Geometry check sheet. Reference: the model listing, model coordinates, mm. A direction names the side the tool comes from. Round coordinates to 2 decimals unless told otherwise and drop trailing zeros. Write each loop counter-clockwise with the first axis right and the second up, starting at its lowest first coordinate (ties: lowest second). Pieces come first, ordered by that corner, then holes. Notation, with made-up numbers: M 78,80.5 L 115,80.5 A13 cw 115,91.5 Z; hole C 3,-38.5 d10. An arc over 180 degrees is marked long. Put each result on its own line as item: value. Start each with the question number.
(1) Material ranges on probe 1 along Y at (x, z) = (-19.5, 26.5); probe 2 along Y at (x, z) = (8.5, 14.5); probe 3 along Z at (x, y) = (-68, 3), recorded low to high.
(2) Section check C-C on y = 19.5. Record the cut outline in (x, z).
(3) Section check D-D on y = -3.5. Record the cut outline in (x, z), then the cut area to 3 significant figures.
(4) Gauge pin test, flat ends, axial feed: pin 1 (9 mm diameter, centred on x = -21, y = -0.5, fed in from +Z); pin 2 (19 mm diameter, centred on x = -26, z = 25, fed in from -Y); pin 3 (13.5 mm diameter, centred on x = 30, y = -71, fed in from +Z). Record the tip position at first contact, or that the pin passes through.
(5) Section check B-B on x = 63. Record the cut outline in (y, z).
(6) Tool access check on faces 1 (the flat face through (-1, -53, 32.545)), 2 (the flat face through (2, -68, 15.158)), 3 (the flat face through (2, 4.999, 23)). Record the directions out of +Z, -Z, +X, -X, +Y, -Y that give a thin tool (end or side, any length) a straight path to the whole face; none if there is none.
(7) Section check A-A on z = 19.5. Record the cut outline in (x, y), then the cut area to 3 significant figures.
from build123d import *

# Parameters (mm, degrees)
F0_W     = 153.3627957106
F0_H     = 90.0560617447
F1_DEPTH = 76.6826
F2_W     = 17.0374948467
F2_H     = 17.3870613798
F2_W_2   = 19.1703476012
F2_H_2   = 18.2787058875
F2_W_3   = 17.8328882903
F2_W_4   = 17.3870567232
F2_H_3   = 19.1703503951
F2_W_5   = 17.8328789771
F2_H_4   = 17.832884565
F3_DEPTH = 228.6


with BuildPart() as f1:
    # F0 (on Front) → F1 (new body, symmetric)
    with BuildSketch(Plane.XZ):
        with Locations((0.4458203912, -12.4830156565)):
            Rectangle(F0_W, F0_H)
    extrude(amount=F1_DEPTH, both=True)

    # F2 (on face) → F3 (cut)
    with BuildSketch(Plane.YZ.offset(77.1272182465)):
        with Locations((-68.1638525767, 23.8514845259)):
            Rectangle(F2_W, F2_H)
        with Locations((-35.7936229557, 23.4056622721)):
            Rectangle(F2_W_2, F2_H_2)
        with Locations((-3.9173448458, 23.4056622721)):
            Rectangle(F2_W_3, F2_H_2)
        with Locations((26.1756433174, 22.9598400183)):
            Rectangle(F2_W_4, F2_H_3)
        with Locations((61.172677204, 23.6285729334)):
            Rectangle(F2_W_5, F2_H_4)
    extrude(amount=-F3_DEPTH, mode=Mode.SUBTRACT)


solid = f1.part
Answers follow:
1. probe 1: y = -59.65 to -45.38, -26.21 to -12.83, 5 to 17.48, 34.87 to 52.26, 70.09 to 76.68
1. probe 2: y = -76.68 to -45.38, -26.21 to -12.83, 5 to 17.48, 34.87 to 76.68
1. probe 3: z = -57.51 to 14.27
2. outline: M -76.24,-57.51 L 77.13,-57.51 L 77.13,13.37 L -76.24,13.37 Z
3. outline: M -76.24,-57.51 L 77.13,-57.51 L 77.13,14.27 L -76.24,14.27 Z
3. area: 11,000 mm^2
4. pin 1: stops at z = 14.27
4. pin 2: stops at y = -59.65
4. pin 3: stops at z = 15.16
5. outline: M -76.68,-57.51 L 76.68,-57.51 L 76.68,32.55 L 70.09,32.55 L 70.09,14.71 L 52.26,14.71 L 52.26,32.55 L 34.87,32.55 L 34.87,13.37 L 17.48,13.37 L 17.48,32.55 L 5,32.55 L 5,14.27 L -12.83,14.27 L -12.83,32.55 L -26.21,32.55 L -26.21,14.27 L -45.38,14.27 L -45.38,32.55 L -59.65,32.55 L -59.65,15.16 L -76.68,15.16 Z
6. face 1: +Z, +X, -X, +Y, -Y
6. face 2: +Z, +X, -X, -Y
6. face 3: +Z, +X, -X
7. outline: M -76.24,-59.65 L 77.13,-59.65 L 77.13,-45.38 L -76.24,-45.38 Z; M -76.24,-26.21 L 77.13,-26.21 L 77.13,-12.83 L -76.24,-12.83 Z; M -76.24,5 L 77.13,5 L 77.13,17.48 L -76.24,17.48 Z; M -76.24,34.87 L 77.13,34.87 L 77.13,52.26 L -76.24,52.26 Z; M -76.24,70.09 L 77.13,70.09 L 77.13,76.68 L -76.24,76.68 Z
7. area: 9,830 mm^2
